Verification items for the finished model (mm, model axes). Give positions to 0.01 mm unless a question says otherwise; leave off trailing zeros. Loops run counter-clockwise (first coordinate to the right, second up) from the corner with the lowest first, then second, coordinate; pieces in that order, holes last. Notation, with made-up numbers: M 23,79 L 53,79 A4 ccw 53,86 Z; hole C 34.5,0.25 d6. An arc over 180 degrees is marked long. Answer in a Markdown table with one row per item.
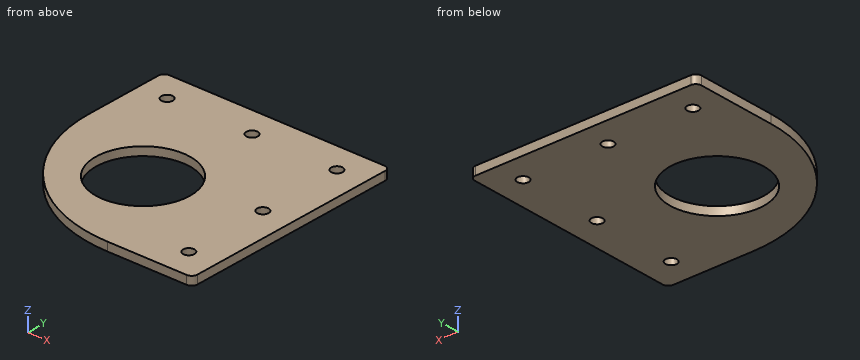
```python
from build123d import *

# Parameters (mm, degrees)
SKETCH_R   = 16.5
SKETCH_R_2 = 2
PAD_DEPTH  = 3
FILLET_R   = 2


with BuildPart() as part:
    # Sketch → Pad (new body)
    with BuildSketch(Plane.XY):
        with BuildLine():
            Line((30, 0), (30, -49.834524))
            Line((30, -49.834524), (0, -49.834524))
            ThreePointArc((-49.834524, 0), (-35.23833, -35.23833), (0, -49.834524))
            Line((-49.834524, 0), (-49.834524, 20))
            Line((-49.834524, 20), (-49.834524, 30))
            Line((-49.834524, 30), (30, 30))
            Line((30, 30), (30, 0))
        make_face()
        with Locations((-16.5, -16.5)):
            Circle(SKETCH_R, mode=Mode.SUBTRACT)
        with Locations((-39.834524, 20)):
            Circle(SKETCH_R_2, mode=Mode.SUBTRACT)
        with Locations((-9.917262, 20)):
            Circle(SKETCH_R_2, mode=Mode.SUBTRACT)
        with Locations((20, 20)):
            Circle(SKETCH_R_2, mode=Mode.SUBTRACT)
        with Locations((20, -9.917262)):
            Circle(SKETCH_R_2, mode=Mode.SUBTRACT)
        with Locations((20, -39.834524)):
            Circle(SKETCH_R_2, mode=Mode.SUBTRACT)
    extrude(amount=PAD_DEPTH)

    # Fillet
    fillet_edges = [part.edges().sort_by_distance(p)[0] for p in [
        (30, -49.834524, 1.5),
        (30, 30, 1.5),
        (-49.834524, 30, 1.5),
    ]]
    fillet(fillet_edges, radius=FILLET_R)


solid = part.part
```
Item 1: Scan lines: L1, parallel to Y at x = 20, z = 1.9; L2, parallel to X at y = 21.5, z = 0.8; L3, parallel to X at y = -21, z = 0.95. Record each from-to range of solid material in increasing order. Write a range as [from, to].
Reported:
| item | result |
|---|---|
| L1 | y = [-49.83, -41.83], [-37.83, -11.92], [-7.92, 18], [22, 30] |
| L2 | x = [-49.83, -41.16], [-38.51, -11.24], [-8.59, 18.68], [21.32, 30] |
| L3 | x = [-45.19, -32.37], [-0.63, 30] |
Item 2: Sectioned sample at A-A (x = 20). Record the cut outline in (y, z).
Reported:
| item | result |
|---|---|
| outline | M -49.83,0 L -41.83,0 L -41.83,3 L -49.83,3 Z; M -37.83,0 L -11.92,0 L -11.92,3 L -37.83,3 Z; M -7.92,0 L 18,0 L 18,3 L -7.92,3 Z; M 22,0 L 30,0 L 30,3 L 22,3 Z |
Item 3: Go/stop test with flat-tipped pins: pin 1 (3 mm diameter, centred on x = 20, y = 20, fed in from -Z); pin 2 (1 mm diameter, centred on x = -17.5, z = 2, fed in from -Y). Record where each tip stops, or that it passes through.
Reported:
| item | result |
|---|---|
| pin 1 | passes through |
| pin 2 | stops at y = -46.85 |
Item 4: Sectioned sample at D-D (y = -2.5). Record the cut outline in (x, z).
Reported:
| item | result |
|---|---|
| outline | M -49.77,0 L -25.23,0 L -25.23,3 L -49.77,3 Z; M -7.77,0 L 30,0 L 30,3 L -7.77,3 Z |
Item 5: Sectioned sample at C-C (z = 1.05). Record the cut outline in (x, y).
Reported:
| item | result |
|---|---|
| outline | M -49.83,0 A49.83 ccw 0,-49.83 L 28,-49.83 A2 ccw 30,-47.83 L 30,28 A2 ccw 28,30 L -47.83,30 A2 ccw -49.83,28 Z; hole C -39.83,20 d4; hole C -16.5,-16.5 d33; hole C -9.92,20 d4; hole C 20,-39.83 d4; hole C 20,-9.92 d4; hole C 20,20 d4 |
